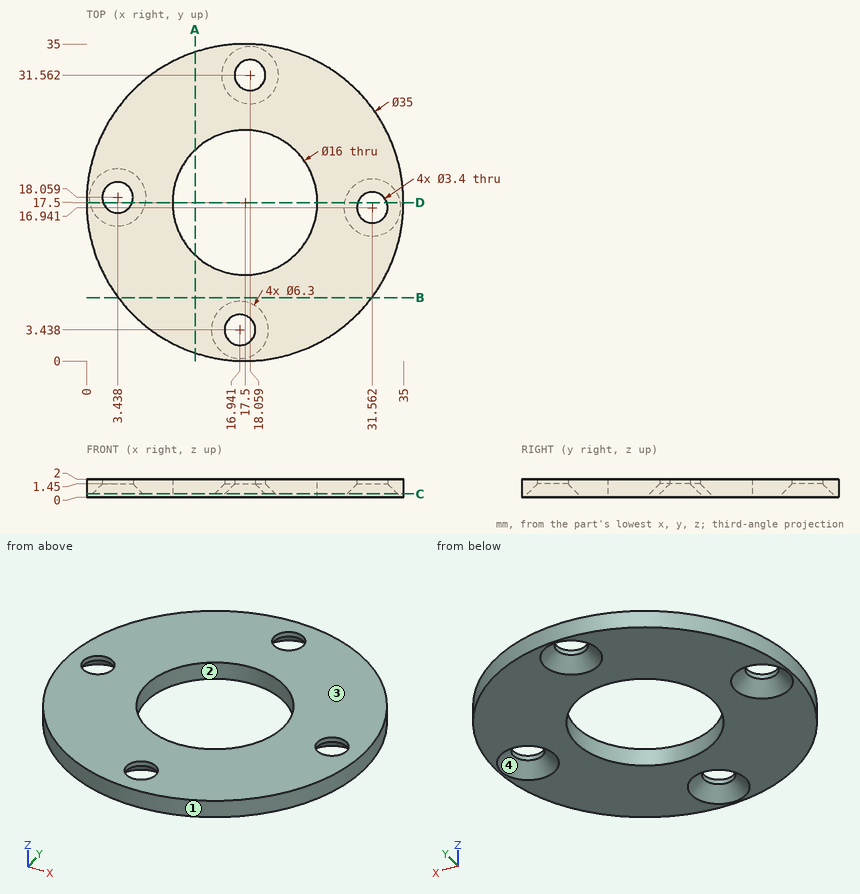
Verification items for this drawing (mm, ordinates from the low corner). Coordinates: 2 decimals unless noted, no trailing zeros. Loops run counter-clockwise (first coordinate to the right, second up) from the corner with the lowest first, then second, coordinate; pieces in that order, holes last.
Item 1: Sectioned sample at A-A, the plane x = 12. Record the boundary of the cut face in (y, z), then the cut area to 3 significant figures.
Item 2: Sectioned sample at C-C, the plane z = 0.35. Record the boundary of the cut face in (x, y).
Item 3: Thickness scan on line 1 (Y direction, x = 17.5, z = 0.7); line 2 (X direction, y = 18, z = 0.9) (1 decimal); line 3 (Y direction, x = 32, z = 1.8). Record the ranges inside material, lowest first.
Item 4: Sectioned sample at D-D, the plane y = 17.5. Count the separate pieces of the cut face and the enclosed holes in it, then the cut area to 3 significant figures.
Item 5: Release check for a two-part mould opening along Y. For the marked faces 1, 2, 3 and 4 record: released by +Y, released by -Y, zero draft, split by the parting line, or undercut.
Item 6: Sectioned sample at B-B, the plane y = 7. Record the boundary of the cut face in (x, z), then the cut area to 3 significant figures.
Check result:
1. outline: (0.89, 0) - (11.69, 0) - (11.69, 2) - (0.89, 2) - close; (23.31, 0) - (34.11, 0) - (34.11, 2) - (23.31, 2) - close
1. area: 43.2 mm2
2. outline: circle Ø35 at (17.5, 17.5); hole circle Ø5.6 at (3.44, 18.06); hole circle Ø16 at (17.5, 17.5); hole circle Ø5.6 at (16.94, 3.44); hole circle Ø5.6 at (18.06, 31.56); hole circle Ø5.6 at (31.56, 16.94)
3. line 1: y = 0 to 1.05, 5.82 to 9.5, 25.5 to 29.18, 33.95 to 35
3. line 2: x = 0 to 1.2, 5.7 to 9.5, 25.5 to 29.6, 33.5 to 35
3. line 3: y = 7.7 to 15.3, 18.58 to 27.3
4. separate pieces: 4
4. enclosed holes: 0
4. area: 20.8 mm2
5. face 1: split by the parting line
5. face 2: undercut
5. face 3: zero draft
5. face 4: undercut
6. outline: (3.5, 0) - (31.5, 0) - (31.5, 2) - (3.5, 2) - close
6. area: 56.0 mm2
